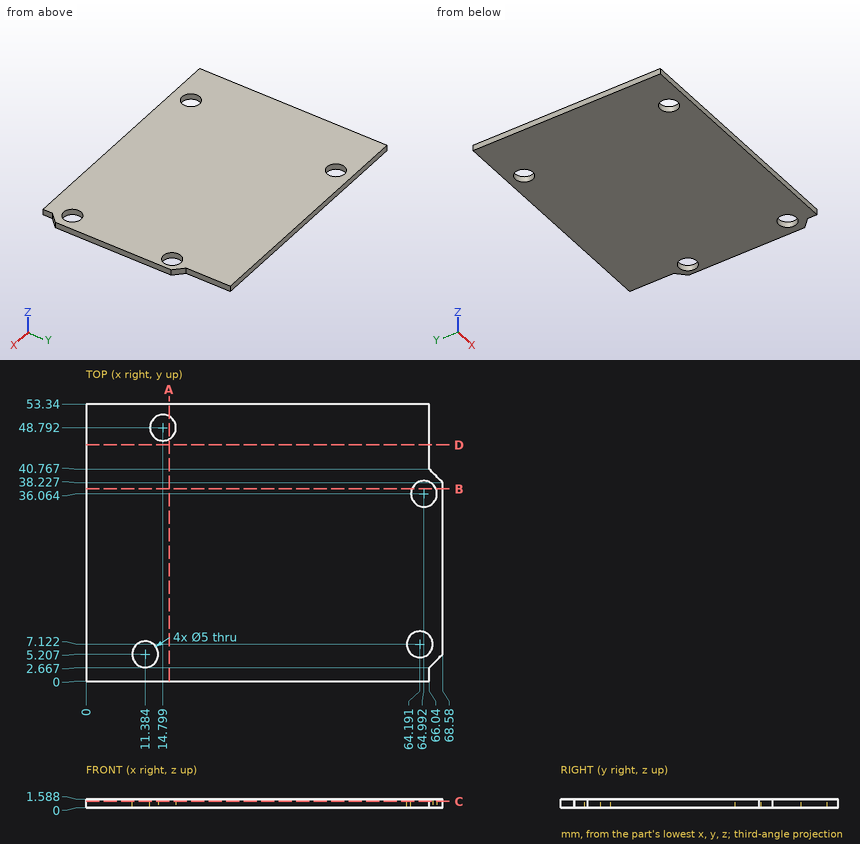
Input: dimensioned drawing with shaded views. Units: mm. Origin: part minimum x, y, z. Round coordinates to 2 decimals unless told otherwise and drop trailing zeros. Loops run counter-clockwise (first coordinate to the right, second up) from the corner with the lowest first, then second, coordinate; pieces in that order, holes last. Notation, with made-up numbers: (16, -34.75) -> (35, -34.75) arc R17 cw to (35, -1.75) -> close; hole circle Ø11 at (40.25, 12.5). An arc over 180 degrees is marked (long way). Answer as a JSON object with one key per item and string values. Group by question number.
1) Section query C-C on z = 1.2. Output: boundary loops of the cut face in (x, y) (1 decimal).
2) Pin query (flat end, axial travel): pin 1 (0.5 mm diameter, centred on y = 2, z = 1, fed in from +X). Return the tip coordinate at first contact, or that it passes through.
3) Section query B-B on y = 37. Output: boundary loops of the cut face in (x, z) (1 decimal).
4) Section query A-A on x = 16. Output: boundary loops of the cut face in (y, z) (1 decimal).
5) Section query D-D on y = 45.5. Output: boundary loops of the cut face in (x, z), plus the area to 3 significant figures.
6) Ray query, L1, parallel to Y at x = 13, z = 0.4 (1 decimal); L2, parallel to X at y = 6.5, z = 1 (1 decimal); L3, parallel to Y at x = 65.5, z = 1.25 (1 decimal). Return the intervals inside material, ascending.
Reply:
{
 "1": {"outline": "(0, 0) -> (66, 0) -> (66, 2.7) -> (68.6, 5.2) -> (68.6, 38.2) -> (66, 40.8) -> (66, 53.3) -> (0, 53.3) -> close; hole circle Ø5 at (11.4, 5.2); hole circle Ø5 at (14.8, 48.8); hole circle Ø5 at (64.2, 7.1); hole circle Ø5 at (65, 36.1)"},
 "2": {"pin 1": "stops at x = 66.04"},
 "3": {"outline": "(0, 0) -> (62.7, 0) -> (62.7, 1.6) -> (0, 1.6) -> close; (67.3, 0) -> (68.6, 0) -> (68.6, 1.6) -> (67.3, 1.6) -> close"},
 "4": {"outline": "(0, 0) -> (46.6, 0) -> (46.6, 1.6) -> (0, 1.6) -> close; (51, 0) -> (53.3, 0) -> (53.3, 1.6) -> (51, 1.6) -> close"},
 "5": {"outline": "(0, 0) -> (66.04, 0) -> (66.04, 1.59) -> (0, 1.59) -> close", "area": "105 mm2"},
 "6": {"L1": "y = 0 to 3.3, 7.1 to 47.1, 50.5 to 53.3", "L2": "x = 0 to 9.2, 13.5 to 61.8, 66.6 to 68.6", "L3": "y = 0 to 5, 9.3 to 33.6, 38.5 to 53.3"}
}
